The listing builds one solid part. Answer for the finished solid, in the listing's coordinates (mm). Face numbers are marked on the shaded views. Give positions to 0.01 mm unless a question says otherwise; leave off trailing zeros. Write each loop counter-clockwise with the first axis right and the second up, starting at its lowest first coordinate (ties: lowest second). Pieces come first, ordered by that corner, then holes. Notation, with made-up numbers: (88, 52.5) - (109, 52.5) arc R23 ccw to (109, 71.5) - close; hole circle Ø2 at (57, 54). An arc over 180 degrees is marked (long way). Answer as CSV lines item,"result". Start each with the question number.
(1) Each of these flat-tipped pins is pushed along its axis until it touches: pin 1 Ø3 at (y, z) = (-3.5, -0.5) entering from -X; pin 2 Ø2 at (x, z) = (1.5, -2) entering from -Y; pin 3 Ø1 at (x, z) = (1.5, -1.5) entering from +Y; pin 4 Ø5.5 at (x, y) = (0, 0) entering from -Z. Where does it stop, or does it pass through?
(2) Find section B-B (x = 0). Write down the section's boundary in (y, z) (3 decimals), then the cut area to 3 significant figures.
(3) Find section A-A (y = 0). Write down the section's boundary in (x, z) (3 decimals).
(4) Straight lines are drawn through the part: probe 1 along X at (y, z) = (0, 1.25) (3 decimals); probe 2 along X at (y, z) = (-2.25, -3.5); probe 3 along Y at (x, z) = (1.25, -1.5). For each, find the intervals that lie inside material, in ascending order.
(5) For a pull along Y with two mould halves and no side action, classify the marked faces 1, 2 and 3 as pulls with the +Y half, pulls with the -Y half, needs draft (parallel to the pull), parting line crosses it, or undercut.
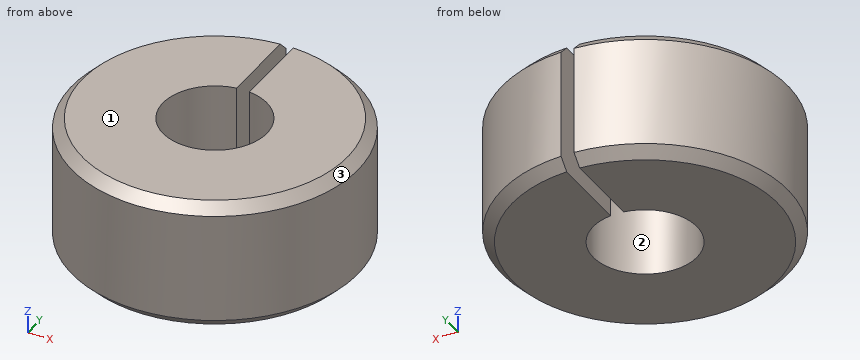
from build123d import *

# Parameters (mm, degrees)
EXTRUSION_DEPTH = 3.96875
CHAMFER1_SIZE   = 0.635


with BuildPart() as part:
    # profile → extrusion (new body, symmetric)
    with BuildSketch(Plane.XY):
        with BuildLine():
            Line((-0.396875, 3.150097655), (-0.396875, 8.72222545))
            ThreePointArc((-0.396875, 8.72222545), (0, -8.73125), (0.396875, 8.72222545))
            Line((0.396875, 8.72222545), (0.396875, 3.150097655))
            ThreePointArc((0.396875, 3.150097655), (0, -3.175), (-0.396875, 3.150097655))
        make_face()
    extrude(amount=EXTRUSION_DEPTH, both=True)

    # Chamfer1
    chamfer1_edges = [part.edges().sort_by_distance(p)[0] for p in [
        (0, -8.73125, 3.96875),
        (0, -8.73125, -3.96875),
    ]]
    chamfer(chamfer1_edges, length=CHAMFER1_SIZE)


solid = part.part
Result set:
1,pin 1,"x = -8.5"
1,pin 2,"y = -8.72"
1,pin 3,"y = 8.67"
1,pin 4,"through"
2,outline,"(-8.731, -3.334) - (-8.096, -3.969) - (-3.175, -3.969) - (-3.175, 3.969) - (-8.096, 3.969) - (-8.731, 3.334) - close"
2,area,"43.7 mm^2"
3,outline,"(-8.731, -3.334) - (-8.096, -3.969) - (-3.175, -3.969) - (-3.175, 3.969) - (-8.096, 3.969) - (-8.731, 3.334) - close; (3.175, -3.969) - (8.096, -3.969) - (8.731, -3.334) - (8.731, 3.334) - (8.096, 3.969) - (3.175, 3.969) - close"
4,probe 1,"-8.731 to -3.175, 3.175 to 8.731"
4,probe 2,"-8.26 to -2.24, 2.24 to 8.26"
4,probe 3,"-8.64 to -2.92, 2.92 to 8.64"
5,face 1,"needs draft"
5,face 2,"undercut"
5,face 3,"parting line crosses it"
